The model under review builds one solid part; all positions refer to its coordinate system, in mm. A direction names the side the tool comes from. Coordinates: 2 decimals unless noted, no trailing zeros. Loops run counter-clockwise (first coordinate to the right, second up) from the corner with the lowest first, then second, coordinate; pieces in that order, holes last. Notation, with made-up numbers: (69, 55) - (73, 55) arc R13 cw to (73, 61) - close; hole circle Ø2 at (19, -18). An arc over 180 degrees is marked (long way). One line per item, written item: value. Start each with the question number.
1. Insertion check: P1, Ø3, axis at x = 51, z = -4.5, coming from the -Y side. The pin has a flat end and moves straight along its axis. Give the tip position at first contact, or say it passes through.
2. To check wall thickness, follow line 1 (Z direction, x = 16.5, y = -0.5); line 2 (Z direction, x = 26, y = 0.7); line 3 (Y direction, x = 30, z = 6). State the ranges of each line that lie inside material, in increasing order.
3. Mouldability with a two-part tool opening along Z and no side actions: class faces 3 (the face through (68.074, 0.014, 0.429)), 4 (the face through (39.133, 0.044, 5.682)) as +Z half, -Z half, draft (parallel to the pull), parting line (faces both ways), or undercut.
4. We need section A-A, the plane y = 0.35. Give the boundary of the cut face in (x, z).
5. For faces 1 (the face through (39.133, 0.044, -5.682)), 2 (the face through (68.074, 0.014, -0.429)), list the 3-axis set-ups (+Z, -Z, +X, -X, +Y, -Y) from which the entire face can be reached by the end or side of a thin tool; tool diameter is ignored.
from build123d import *

# Parameters (mm, degrees)
F0_R          = 1
F1_ANGLE_BACK = 99
F1_ANGLE      = 198
F2_DEPTH      = 58
F3_DEPTH      = 58


with BuildPart() as f1:
    # F0 (on Top) → F1 (revolve)
    with BuildSketch(Plane.XY, mode=Mode.PRIVATE) as f1_sk:
        Circle(F0_R)
    revolve(f1_sk.sketch.rotate(Axis((9.283, 0.6793318316, 0), (0, 1, 0)), -F1_ANGLE_BACK), axis=Axis((9.283, 0.6793318316, 0), (0, 1, 0)), revolution_arc=F1_ANGLE)

    # F2 (add): a face of the model
    f2_faces = [f1.faces().sort_by_distance(p)[0] for p in [
        (10.735181139, 0, 9.1687108657),
    ]]
    extrude(f2_faces, amount=F2_DEPTH)

    # F3 (add): a face of the model
    f3_faces = [f1.faces().sort_by_distance(p)[0] for p in [
        (10.735181139, 0, -9.1687108657),
    ]]
    extrude(f3_faces, amount=F3_DEPTH)


solid = f1.part
Findings below:
1. P1: y = -0.98
2. line 1: -9.13 to -7.38, 7.38 to 9.13
2. line 2: -7.47 to -6.03, 6.03 to 7.47
2. line 3: -0.99 to 0.99
3. face 3: undercut
3. face 4: undercut
4. outline: (10.88, -10.09) - (68.17, -1.02) - (68.01, 0) - (68.17, 1.02) - (10.88, 10.09) arc R10.22 ccw (long way) to start; hole (10.59, -8.24) - (62.64, 0) - (10.59, 8.24) arc R8.35 ccw (long way) to start
5. face 1: none
5. face 2: +X, +Y, -Y
